Build history of the part. All positions in model axes, mm. A direction names the side the tool comes from. Round coordinates to 2 decimals unless told otherwise and drop trailing zeros. Write each loop counter-clockwise with the first axis right and the second up, starting at its lowest first coordinate (ties: lowest second). Pieces come first, ordered by that corner, then holes.
Item 1: Band-saw the part on C-C, the plane z = 10.75. Write the cut outline in (x, y), then the cut area to 3 significant figures.
Item 2: 3-axis set-ups, long thin cutter, end or side, ignore diameter. For faces 1 (the flat face through (29.21, 38, 9)), 2 (the flat face through (-1.27, 38, 9)), 3 (the cylindrical face through (19.596, 27.284, 9.569)), 4 (the flat face through (14, 53.34, 9)): which of +Z, -Z, +X, -X, +Y, -Y reach the whole face in a straight line?
Item 3: Band-saw the part on D-D, the plane y = -46.5. Write the cut outline in (x, z), then the cut area to 3 significant figures.
Item 4: Band-saw the part on A-A, the plane y = 38.1. Write the cut outline in (x, z), then the cut area to 3 significant figures.
Item 5: Drop flat-ended pins along their axis: pin 1 Ø3 at (x, z) = (15.5, 9) entering from -Y; pin 2 Ø1.5 at (x, z) = (-12, 8.5) entering from -Y; pin 3 Ø5 at (x, z) = (16.5, 10.5) entering from +Y; pin 4 Ø1.9 at (y, z) = (35, 10.5) entering from -X. Give the stop position or say it passes through.
Item 6: Wall check: probe 1 along Y at (x, z) = (13.97, 8); probe 2 along Y at (x, z) = (13.97, 2.5); probe 3 along Z at (x, y) = (-18.5, -65). Give the ranges that are in metal, low to high.
Item 7: Band-saw the part on B-B, the plane x = 13.97. Write the cut outline in (y, z), then the cut area to 3 significant figures.
Item 8: Mould opens along X. For faces 5 (the flat face through (18.4, 46.3, 6.35)), 6 (the flat face through (44.45, -1, 3)), 7 (the flat face through (-1, 1, 6.35)) say: +X half, -X half, draft (parallel to the pull), parting line (faces both ways), or undercut.
```python
from build123d import *

# Parameters (mm, degrees)
F1_DEPTH       = 6.35
F0_W           = 15.24
F0_H           = 15.24
F2_DEPTH       = 12.7
F4_D           = 18.288
F4_CBORE_D     = 24.384
F4_CBORE_DEPTH = 6.35


with BuildPart() as f1:
    # F0 (on Top) → F1 (new body)
    with BuildSketch(Plane.XY):
        Polygon((-44.45, -76.2), (44.45, -76.2), (44.45, 38.1), (29.21, 38.1), (29.21, 22.86), (-1.27, 22.86), (-1.27, 53.34), (13.97, 53.34), (13.97, 76.2), (-44.45, 76.2), align=None)
        Polygon((29.21, 38.1), (44.45, 38.1), (44.45, 76.2), (13.97, 76.2), (13.97, 53.34), (29.21, 53.34), align=None)
    extrude(amount=F1_DEPTH)

    # F0 (on Top) → F2 (join)
    with BuildSketch(Plane.XY):
        Polygon((29.21, 22.86), (29.21, 38.1), (13.97, 38.1), (13.97, 53.34), (-1.27, 53.34), (-1.27, 22.86), align=None)
        with Locations((21.59, 45.72)):
            Rectangle(F0_W, F0_H)
    extrude(amount=F2_DEPTH)

    # F4 (through all)
    with Locations(Plane.XY.offset(12.7)):
        with Locations((13.97, 38.1)):
            CounterBoreHole(F4_D / 2, F4_CBORE_D / 2, F4_CBORE_DEPTH)


solid = f1.part
```
Results:
1. outline: (-1.27, 22.86) - (29.21, 22.86) - (29.21, 53.34) - (-1.27, 53.34) - close; hole circle Ø24.38 at (13.97, 38.1)
1. area: 462 mm2
2. face 1: +Z, +X, +Y, -Y
2. face 2: +Z, -X, +Y, -Y
2. face 3: +Z
2. face 4: +Z, +X, -X, +Y
3. outline: (-44.45, 0) - (44.45, 0) - (44.45, 6.35) - (-44.45, 6.35) - close
3. area: 565 mm2
4. outline: (-44.45, 0) - (4.83, 0) - (4.83, 6.35) - (1.78, 6.35) - (1.78, 12.7) - (-1.27, 12.7) - (-1.27, 6.35) - (-44.45, 6.35) - close; (23.11, 0) - (44.45, 0) - (44.45, 6.35) - (29.21, 6.35) - (29.21, 12.7) - (26.16, 12.7) - (26.16, 6.35) - (23.11, 6.35) - close
4. area: 487 mm2
5. pin 1: stops at y = 22.86
5. pin 2: passes through
5. pin 3: stops at y = 53.34
5. pin 4: stops at x = -1.27
6. probe 1: y = 22.86 to 25.91, 50.29 to 53.34
6. probe 2: y = -76.2 to 28.96, 47.24 to 76.2
6. probe 3: z = 0 to 6.35
7. outline: (-76.2, 0) - (28.96, 0) - (28.96, 6.35) - (25.91, 6.35) - (25.91, 12.7) - (22.86, 12.7) - (22.86, 6.35) - (-76.2, 6.35) - close; (47.24, 0) - (76.2, 0) - (76.2, 6.35) - (53.34, 6.35) - (53.34, 12.7) - (50.29, 12.7) - (50.29, 6.35) - (47.24, 6.35) - close
7. area: 890 mm2
8. face 5: undercut
8. face 6: +X half
8. face 7: draft
